from build123d import *

# Parameters (mm, degrees)
EXTRUDE_1_DEPTH     = 10
SKETCH_2_R          = 7.5
CUT_EXTRUDE_1_DEPTH = 10


with BuildPart() as part:
    # 草图1 → 凸台-拉伸1 (new body)
    with BuildSketch(Plane(origin=(0, 0, 0), x_dir=(1, 0, 0), z_dir=(0, 1, 0))):
        with BuildLine():
            Line((-0.759854477, 9.958566069), (12.573478857, 5.244520861))
            ThreePointArc((12.573478857, 5.244520861), (19.240145523, -4.183569555), (12.573478857, -13.611659971))
            Line((12.573478857, -13.611659971), (-0.759854477, -18.325705179))
            ThreePointArc((-0.759854477, -18.325705179), (-20.759854477, -4.183569555), (-0.759854477, 9.958566069))
        make_face()
    extrude(amount=EXTRUDE_1_DEPTH)

    # 草图2 → 切除-拉伸1 (cut)
    with BuildSketch(Plane(origin=(0, 10, 0), x_dir=(1, 0, 0), z_dir=(0, 1, 0))):
        with Locations(Location((-5.759854477, -4.183569555, 0), (0, 0, 270))):
            Circle(SKETCH_2_R)
    extrude(amount=-CUT_EXTRUDE_1_DEPTH, mode=Mode.SUBTRACT)


solid = part.part
CAD build for the part. Positions are in the model's coordinates, mm. Round coordinates to 2 decimals unless told otherwise and drop trailing zeros. Loops run counter-clockwise (first coordinate to the right, second up) from the corner with the lowest first, then second, coordinate; pieces in that order, holes last. Notation, with made-up numbers: M 51.25,79.25 L 69.25,79.25 A19 ccw 69.25,111.25 Z; hole C -13.75,-17 d11. An arc over 180 degrees is marked long. One line per question, with ' | ' between items. Start each with the question number.
Item 1: Cut at A-A, the plane x = -8. Write the cut outline in (y, z), plus the area to 3 significant figures.
Item 2: Cut at B-B, the plane z = 7. Write the cut outline in (x, y).
Item 3: Two-plate mould, pull along Z, no slides. Class faces 1 (the cylindrical face through (-20.754, 4.93, 4.585)), 2 (the flat face through (6, 4.93, 15.936)), 3 (the cylindrical face through (-13.08, 5.07, 2.56)): pulls with the +Z half, pulls with the -Z half, needs draft (parallel to the pull), parting line crosses it, or undercut.
Item 4: Pin check, flat tips, straight feed: pin 1 Ø3 at (y, z) = (4.5, -4) entering from -X; pin 2 Ø2 at (y, z) = (2, 7) entering from -X; pin 3 Ø3 at (y, z) = (8, 14.5) entering from +X. Stop position of each tip, or through.
Item 5: Cut at C-C, the plane y = 6.25. Write the cut outline in (x, z), plus the area to 3 significant figures.
Item 6: Cut at D-D, the plane z = -8. Write the cut outline in (x, y), plus the area to 3 significant figures.
Item 7: Wall check: line 1 (Z direction, x = -8, y = 1); line 2 (Z direction, x = -5.5, y = 3.5); line 3 (X direction, y = 5.25, z = -2.5). Give the ranges that are in metal, low to high.
Responses:
1) outline: M 0,-10.65 L 10,-10.65 L 10,-2.97 L 0,-2.97 Z; M 0,11.34 L 10,11.34 L 10,19.02 L 0,19.02 Z | area: 153 mm²
2) outline: M -20.49,0 L -12.71,0 L -12.71,10 L -20.49,10 Z; M 1.19,0 L 18.84,0 L 18.84,10 L 1.19,10 Z
3) face 1: parting line crosses it | face 2: pulls with the +Z half | face 3: undercut
4) pin 1: stops at x = -19.19 | pin 2: stops at x = -20.65 | pin 3: stops at x = 13.96
5) outline: M -0.76,-9.96 L 12.57,-5.24 A10 ccw 12.57,13.61 L -0.76,18.33 A15 ccw long Z; hole C -5.76,4.18 d15 | area: 730 mm²
6) outline: M -14.51,0 L 4.78,0 L 4.78,10 L -14.51,10 Z | area: 193 mm²
7) line 1: z = -10.65 to -2.97, 11.34 to 19.02 | line 2: z = -10.81 to -3.31, 11.68 to 19.18 | line 3: x = -19.19 to -9.16, -2.36 to 16.68
